Autodesk Inventor part; units mm, degrees
ref_plane "YZ Plane" through (0, 0, 0) normal (1, 0, 0) x (0, 1, 0)
ref_plane "XZ Plane" through (0, 0, 0) normal (0, 1, 0) x (-1, 0, 0)
ref_plane "XY Plane" through (0, 0, 0) normal (0, 0, 1) x (1, 0, 0)
sketch "Sketch1" plane through (0, 0, 0) normal (0, 0, 1) x (1, 0, 0)
  line L0 (0, 0) -> (110, 0)
  line L1 (110, 0) -> (110, 110)
  line L2 (110, 110) -> (0, 110)
  line L3 (0, 110) -> (0, 0)
  line L4 (0, 0) -> (0, -3)
  line L5 (0, -3) -> (-3, -3)
  line L6 (-3, -3) -> (113, -3)
  line L7 (113, -3) -> (113, 113)
  line L8 (113, 113) -> (-3, 113)
  line L9 (-3, 113) -> (-3, -3)
  dimension "d0" = 110
  dimension "d1" = 110
  dimension "d2" = 3
  dimension "d3" = 3
  dimension "d4" = 116
  dimension "d5" = 116
extrude "Extrusion1" add sketch "Sketch1" along normal blind 4 contours L3 L2 L1 L0
extrude "Extrusion2" add sketch "Sketch1" along normal blind 2
sketch "Sketch2" plane through (0, 0, 4) normal (0, 0, 1) x (1, 0, 0)
  line L0 (0, 0) -> (110, 0)
  line L1 (55, 0) -> (55, 5)
  line L2 (55, 5) -> (10, 5)
  line L3 (10, 5) -> (100, 5)
  line L4 (100, 5) -> (100, 99)
  line L5 (100, 99) -> (10, 99)
  circle A0 centre (10, 99) radius 3.5
  circle A1 centre (100, 99) radius 3.5
  circle A2 centre (100, 5) radius 3.5
  circle A3 centre (10, 5) radius 3.5
  dimension "d10" = 5
  dimension "d11" = 45
  dimension "d12" = 90
  dimension "d13" = 94
  dimension "d14" = 90
  dimension "d15" = 7
  dimension "d16" = 7
  dimension "d17" = 7
  dimension "d18" = 7
extrude "Extrusion3" add sketch "Sketch2" along normal blind 13
sketch "Sketch3" plane through (10, 99, 17) normal (0, 0, 1) x (1, 0, 0)
  circle A0 centre (0, -94) radius 3.5
  circle A1 centre (0, -94) radius 1.75
  circle A2 centre (90, -94) radius 3.5
  circle A3 centre (90, -94) radius 1.75
  circle A4 centre (90, 0) radius 3.5
  circle A5 centre (90, 0) radius 1.75
  circle A6 centre (0, 0) radius 1.75
  point P0 (-10, -99)
  dimension "d21" = 3.5
  dimension "d22" = 3.5
  dimension "d23" = 3.5
  dimension "d24" = 3.5
extrude "Extrusion4" cut sketch "Sketch3" against normal through all contours A1 | A3 | A5 | A6
sketch "Sketch4" plane through (0, 0, 4) normal (0, 0, 1) x (1, 0, 0)
  line L0 (0, 0) -> (110, 0)
  line L1 (55, 0) -> (55, 20)
  line L2 (55, 20) -> (85, 20)
  line L3 (85, 20) -> (85, 80)
  line L4 (85, 80) -> (25, 80)
  line L5 (25, 80) -> (25, 20)
  circle A0 centre (25, 80) radius 1.75
  circle A1 centre (85, 80) radius 1.75
  circle A2 centre (85, 20) radius 1.75
  circle A3 centre (25, 20) radius 1.75
  dimension "d27" = 20
  dimension "d28" = 30
  dimension "d29" = 60
  dimension "d30" = 60
  dimension "d31" = 60
  dimension "d32" = 3.5
  dimension "d33" = 3.5
  dimension "d34" = 3.5
  dimension "d35" = 3.5
extrude "Extrusion5" cut sketch "Sketch4" against normal blind 15
properties part number "nuccase_top"
Could you check a few things on this model? Use its own coordinates, in mm. A direction names the side the tool comes from. Coordinates: 2 decimals unless noted, no trailing zeros. Loops run counter-clockwise (first coordinate to the right, second up) from the corner with the lowest first, then second, coordinate; pieces in that order, holes last.
1. We'd pull the mould along Y, two halves only. Please class faces 1 (the face through (99.62, 3.29, 8.62)), 2 (the face through (101, 7, 17)): released by +Y, released by -Y, zero draft, split by the parting line, or undercut.
2. For P1, Ø1.5, axis at x = 65.5, y = 43.5, coming from the +Z side; P2, Ø3, axis at x = 99.5, z = 14.5, coming from the -Y side; P3, Ø2, axis at x = 100, y = 99, coming from the -Z side; P4, Ø1.6, axis at y = 54, z = 3, coming from the -X side, each with a flat end and sliding along its axis, tell me the tip position at first contact or that it passes through.
3. Imagine slicing it at A-A (y = 80). Please give me the cut outline in (x, z), and give its area (3 significant figures).
4. For faces 3 (the face through (103.233, 100.341, 10.409)), 4 (the face through (54, 56, 0)), which set-ups out of +Z, -Z, +X, -X, +Y, -Y let a thin tool reach every point of the face, with its end or its side?
5. Imagine slicing it at B-B (x = 25). Please give me the cut outline in (y, z).
6. I need wall thicknesses on L1, parallel to Y at x = 100, z = 6.25; L2, parallel to Y at x = 25, z = 2.5; L3, parallel to Y at x = 85, z = 0.85. Which ranges of each line are inside material? Lowest first, please.
7. Imagine slicing it at C-C (x = 100). Please give me the cut outline in (y, z), and give its area (3 significant figures).
Computed values:
1. face 1: undercut
1. face 2: zero draft
2. P1: stops at z = 4
2. P2: stops at y = 1.5
2. P3: passes through
2. P4: stops at x = 0
3. outline: (-3, 0) - (23.25, 0) - (23.25, 4) - (0, 4) - (0, 2) - (-3, 2) - close; (26.75, 0) - (83.25, 0) - (83.25, 4) - (26.75, 4) - close; (86.75, 0) - (113, 0) - (113, 2) - (110, 2) - (110, 4) - (86.75, 4) - close
3. area: 424 mm2
4. face 3: +Z
4. face 4: -Z, +X, -X, +Y, -Y
5. outline: (-3, 0) - (18.25, 0) - (18.25, 4) - (0, 4) - (0, 2) - (-3, 2) - close; (21.75, 0) - (78.25, 0) - (78.25, 4) - (21.75, 4) - close; (81.75, 0) - (113, 0) - (113, 2) - (110, 2) - (110, 4) - (81.75, 4) - close
6. L1: y = 1.5 to 3.25, 6.75 to 8.5, 95.5 to 97.25, 100.75 to 102.5
6. L2: y = 0 to 18.25, 21.75 to 78.25, 81.75 to 110
6. L3: y = -3 to 18.25, 21.75 to 78.25, 81.75 to 113
7. outline: (-3, 0) - (3.25, 0) - (3.25, 17) - (1.5, 17) - (1.5, 4) - (0, 4) - (0, 2) - (-3, 2) - close; (6.75, 0) - (97.25, 0) - (97.25, 17) - (95.5, 17) - (95.5, 4) - (8.5, 4) - (8.5, 17) - (6.75, 17) - close; (100.75, 0) - (113, 0) - (113, 2) - (110, 2) - (110, 4) - (102.5, 4) - (102.5, 17) - (100.75, 17) - close
7. area: 515 mm2
